from build123d import *

# Parameters (mm, degrees)
BOSS_EXTRUDE1_DEPTH = 8
SKETCH2_R           = 2.5
CUT_EXTRUDE1_DEPTH  = 8
SKETCH3_R           = 3.5
CUT_EXTRUDE2_DEPTH  = 3


with BuildPart() as part:
    # Sketch1 → Boss-Extrude1 (new body)
    with BuildSketch(Plane(origin=(0, 0, 0), x_dir=(1, 0, 0), z_dir=(0, 1, 0))):
        Polygon((4.330127019, 2.5), (0, 5), (-4.330127019, 2.5), (-4.330127019, -2.5), (0, -5), (4.330127019, -2.5), align=None)
    extrude(amount=BOSS_EXTRUDE1_DEPTH)

    # Sketch2 → Cut-Extrude1 (cut)
    with BuildSketch(Plane(origin=(0, 8, 0), x_dir=(1, 0, 0), z_dir=(0, 1, 0))):
        with Locations(Location((0, 0.5, 0), (0, 0, 270))):
            Circle(SKETCH2_R)
    extrude(amount=-CUT_EXTRUDE1_DEPTH, mode=Mode.SUBTRACT)

    # Sketch3 → Cut-Extrude2 (cut)
    with BuildSketch(Plane(origin=(0, 8, 0), x_dir=(1, 0, 0), z_dir=(0, 1, 0))):
        Polygon((-4.330127019, 2.5), (-4.330127019, -2.5), (0, -5), (4.330127019, -2.5), (4.330127019, 2.5), (0, 5), align=None)
        with Locations(Location((0, 0, 0), (0, 0, 270))):
            Circle(SKETCH3_R, mode=Mode.SUBTRACT)
    extrude(amount=-CUT_EXTRUDE2_DEPTH, mode=Mode.SUBTRACT)


solid = part.part
Input: part model. Units: mm. Frame: model coordinates. A direction names the side the tool comes from. Give positions to 0.01 mm unless a question says otherwise; leave off trailing zeros. Order: outer loops, then holes, each group sorted by start corner. A loop starts at its lowest first (then second) coordinate and runs counter-clockwise, first axis right, second up. Notation, with made-up numbers: M 74,15 L 131,15 A19 cw 131,20 Z; hole C 10,-23.5 d9. An arc over 180 degrees is marked long. Answer as a JSON object with one key per item and string values.
1. Cut plane A-A, the plane x = 1. Output: boundary loops of the cut face in (y, z).
Result sheet:
{"outline": "M 0,-4.42 L 5,-4.42 L 5,-3.35 L 8,-3.35 L 8,-2.79 L 0,-2.79 Z; M 0,1.79 L 8,1.79 L 8,3.35 L 5,3.35 L 5,4.42 L 0,4.42 Z"}
2. Reachability of faces 4 (the flat face through (2, 8, 2)), 5 (the flat face through (1.6, 5, 3.3)) from +Z, -Z, +X, -X, +Y, -Y: full face, straight path, thin tool, end or side. Return the list, or none.
Result sheet:
{"face 4": "+Z, -Z, +X, -X, +Y", "face 5": "+Y"}
3. Cut plane D-D, the plane z = -3.25. Output: boundary loops of the cut face in (x, y), and give its area (3 significant figures).
Result sheet:
{"outline": "M -3.03,0 L 3.03,0 L 3.03,5 L 1.3,5 L 1.3,8 L -1.3,8 L -1.3,5 L -3.03,5 Z", "area": "38.1 mm²"}
4. Ray query, line 1 (X direction, y = 4.75, z = -0.5); line 2 (X direction, y = 7.75, z = -2); line 3 (Y direction, x = 0.25, z = -4). Return the intervals inside material, ascending. Write a range as [from, to].
Result sheet:
{"line 1": "[-4.33, -2.5], [2.5, 4.33]", "line 2": "[-2.87, -2], [2, 2.87]", "line 3": "[0, 5]"}
5. Pull-direction query (Z, two-part tool) for faces 1 (the flat face through (-0.1, 0, 2.2)), 2 (the cylindrical face through (-2.44, 4.06, -1.04)), 3 (the cylindrical face through (-3.417, 6.521, -0.759)); classes: +Z half, -Z half, draft (parallel to the pull), parting line (faces both ways), or undercut.
Result sheet:
{"face 1": "draft", "face 2": "undercut", "face 3": "parting line"}
6. Cut plane C-C, the plane y = 1.5. Output: boundary loops of the cut face in (x, z), and give its area (3 significant figures).
Result sheet:
{"outline": "M -4.33,-2.5 L 0,-5 L 4.33,-2.5 L 4.33,2.5 L 0,5 L -4.33,2.5 Z; hole C 0,-0.5 d5", "area": "45.3 mm²"}
7. First-contact query: P1, Ø4, axis at x = 0, z = -0.5, coming from the +Y side; P2, Ø2, axis at x = -2.5, y = 1, coming from the -Z side. Flat tips, straight axial feed; report the tip coordinate or a pass-through.
Result sheet:
{"P1": "through", "P2": "z = -4.13"}
8. Cut plane B-B, the plane z = -0.5. Output: boundary loops of the cut face in (x, y).
Result sheet:
{"outline": "M -4.33,0 L -2.5,0 L -2.5,8 L -3.46,8 L -3.46,5 L -4.33,5 Z; M 2.5,0 L 4.33,0 L 4.33,5 L 3.46,5 L 3.46,8 L 2.5,8 Z"}
